Here's how the part is built. I have some questions about the finished solid (model axes, mm). A direction names the side the tool comes from. Round coordinates to 2 decimals unless told otherwise and drop trailing zeros. Write each loop counter-clockwise with the first axis right and the second up, starting at its lowest first coordinate (ties: lowest second). Pieces come first, ordered by that corner, then holes. Notation, with made-up numbers: (11.25, 43.5) -> (20.25, 43.5) arc R18 cw to (20.25, 63.5) -> close; hole circle Ø2 at (74, 2). An arc over 180 degrees is marked (long way). Put each result on its own line as item: value. Start each with the question number.
1) Which directions (+Z, -Z, +X, -X, +Y, -Y) give clear straight access to the entire face, cutting with the end or side of a thin tool? Please do faces 5 (the flat face through (-2, 20, 4)), 6 (the flat face through (2.5, -4, 0)), 7 (the cylindrical face through (-0.878, 12.605, 3.954)), 8 (the flat face through (0, -4, 2.5)).
2) If I drill on line 1 along Z through (x, y) = (0, 15); line 2 along Z through (x, y) = (-2, 15), over which ranges is the centre line in solid material (lowest first)? Write a range as [from, to].
3) Will these pins go through, and if not, where does the flat tip stop? P1, Ø1, axis at y = 5, z = 2.5, coming from the -X side; P2, Ø2, axis at y = 4, z = -2.5, coming from the -X side; P3, Ø5, axis at x = -3, y = 13, coming from the -Z side.
4) We'd pull the mould along X, two halves only. Please class faces 1 (the cylindrical face through (2.215, -9.699, -0.035)), 2 (the flat face through (0, 5, 0)), 3 (the flat face through (0, -4, -2.5)), 4 (the flat face through (-2.5, -4, 0)): released by +X, released by -X, zero draft, split by the parting line, or undercut.
5) I want a section at D-D, the plane y = -3. List the corners of the cut face in (x, z) for me.
6) I want a section at A-A, the plane z = 0. List the corners of the cut face in (x, y) for me, then the cut area to 3 significant figures.
7) I want a section at C-C, the plane y = 10.5. List the corners of the cut face in (x, z) for me.
8) I want a section at B-B, the plane x = 0. List the corners of the cut face in (y, z) for me.
Autodesk Inventor part; units mm, degrees
ref_plane "YZ Plane" through (0, 0, 0) normal (1, 0, 0) x (0, 1, 0)
ref_plane "XZ Plane" through (0, 0, 0) normal (0, 1, 0) x (-1, 0, 0)
ref_plane "XY Plane" through (0, 0, 0) normal (0, 0, 1) x (1, 0, 0)
sketch "Sketch1" plane through (0, 0, 0) normal (0, 1, 0) x (-1, 0, 0)
  circle A0 centre (0, 0) radius 5.5
  line L0 (2.5, 2.5) -> (-2.5, 2.5)
  line L1 (-2.5, 2.5) -> (-2.5, -2.5)
  line L2 (-2.5, -2.5) -> (2.5, -2.5)
  line L3 (2.5, -2.5) -> (2.5, 2.5)
  line L4 (2.5, 2.5) -> (-2.5, -2.5) construction
  line L5 (-2.5, 2.5) -> (2.5, -2.5) construction
  dimension "d0" = 11
  dimension "d3" = 5
  dimension "d4" = 5
extrude "Extrusion1" add sketch "Sketch1" along normal blind 10 contours A0 | L3 L2 L1 L0
extrude "Extrusion2" add sketch "Sketch1" against normal blind 10 contours L3 L2 L1 L0
fillet "Fillet1" radius 1 4 edges at (0, -10, -2.5) (-2.5, -10, 0) (0, -10, 2.5) (2.5, -10, 0)
fillet "Fillet2" radius 1 1 edges at (5.5, 0, 0)
sketch "Sketch2" plane through (0, 10, 0) normal (0, 1, 0) x (1, 0, 0)
  circle A0 centre (0, 0) radius 4.05
  circle A1 centre (0, 0) radius 5.5
  dimension "d9" = 8.1
  dimension "d10" = 11
extrude "Extrusion3" cut sketch "Sketch2" against normal blind 5 contours A0
sketch "Sketch3" plane through (0, 10, 0) normal (0, 1, 0) x (1, 0, 0)
  point P0 (0, 0)
sketch "Sketch4" plane through (0, 10, 0) normal (0, 1, 0) x (1, 0, 0)
  circle A0 centre (0, 0) radius 5.5
  circle A1 centre (0, 0) radius 4.05
  dimension "d13" = 11
extrude "Extrusion4" add sketch "Sketch4" along normal blind 10
properties part number "nut a"
Findings:
1. face 5: +Z, -Z, +X, -X, +Y
1. face 6: +Z, -Z, +X, -Y
1. face 7: +Y
1. face 8: +Z, +X, -X, -Y
2. line 1: z = [-5.5, -4.05], [4.05, 5.5]
2. line 2: z = [-5.12, -3.52], [3.52, 5.12]
3. P1: stops at x = -5.12
3. P2: stops at x = -5.29
3. P3: stops at z = -5.48
4. face 1: released by +X
4. face 2: undercut
4. face 3: zero draft
4. face 4: released by -X
5. outline: (-2.5, -2.5) -> (2.5, -2.5) -> (2.5, 2.5) -> (-2.5, 2.5) -> close
6. outline: (-5.5, 1) arc R1 ccw to (-4.5, 0) -> (-2.5, 0) -> (-2.5, -9) arc R1 ccw to (-1.5, -10) -> (1.5, -10) arc R1 ccw to (2.5, -9) -> (2.5, 0) -> (4.5, 0) arc R1 ccw to (5.5, 1) -> (5.5, 20) -> (4.05, 20) -> (4.05, 5) -> (-4.05, 5) -> (-4.05, 20) -> (-5.5, 20) -> close
6. area: 148 mm2
7. outline: circle Ø11 at (0, 0); hole circle Ø8.1 at (0, 0)
8. outline: (-10, -1.5) arc R1 ccw to (-9, -2.5) -> (0, -2.5) -> (0, -4.5) arc R1 ccw to (1, -5.5) -> (20, -5.5) -> (20, -4.05) -> (5, -4.05) -> (5, 4.05) -> (20, 4.05) -> (20, 5.5) -> (1, 5.5) arc R1 ccw to (0, 4.5) -> (0, 2.5) -> (-9, 2.5) arc R1 ccw to (-10, 1.5) -> close
